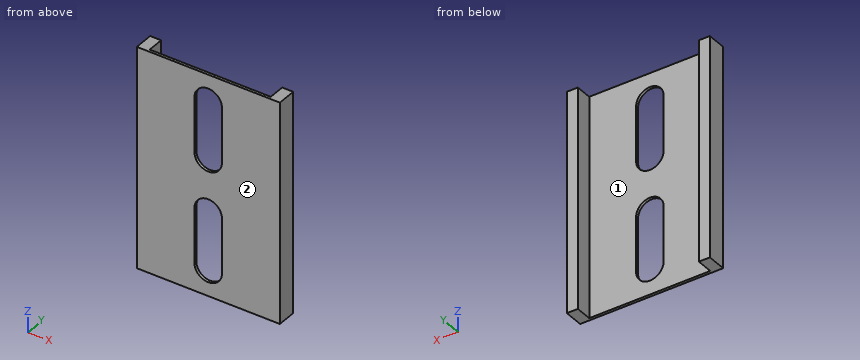
from build123d import *

# Parameters (mm, degrees)
F1_DEPTH = 400
F3_DEPTH = 25


with BuildPart() as f1:
    # F0 (on Top) → F1 (new body)
    with BuildSketch(Plane.XY):
        Polygon((-130, 17.5), (-130, -17.5), (130, -17.5), (130, 17.5), (110, 17.5), (110, -12.5), (-110, -12.5), (-110, 17.5), align=None)
    extrude(amount=F1_DEPTH)

    # F2 (on face) → F3 (cut)
    with BuildSketch(Plane.XZ.offset(17.5)):
        with BuildLine():
            Line((-25.221969, 350), (-25.221969, 250))
            ThreePointArc((-25.221969, 250), (-0.221969, 225), (24.778031, 250))
            Line((24.778031, 250), (24.778031, 350))
            ThreePointArc((24.778031, 350), (-0.221969, 375), (-25.221969, 350))
        make_face()
        with BuildLine():
            Line((24.778031, 50), (24.778031, 150))
            ThreePointArc((24.778031, 150), (-0.221969, 175), (-25.221969, 150))
            Line((-25.221969, 150), (-25.221969, 50))
            ThreePointArc((-25.221969, 50), (-0.221969, 25), (24.778031, 50))
        make_face()
    extrude(amount=-F3_DEPTH, mode=Mode.SUBTRACT)


solid = f1.part
Input: part model. Units: mm. Frame: model coordinates. Face numbers are marked on the shaded views. Coordinates: 2 decimals unless noted, no trailing zeros. Order: outer loops, then holes, each group sorted by start corner. A loop starts at its lowest first (then second) coordinate and runs counter-clockwise, first axis right, second up.
1. Cut plane B-B, the plane y = -2.5. Return loops of the section in (x, z), plus the area to 3 significant figures.
Checked values:
outline: (-130, 0) - (-110, 0) - (-110, 400) - (-130, 400) - close; (110, 0) - (130, 0) - (130, 400) - (110, 400) - close
area: 16,000 mm2
2. Contact query for a flat-ended pin moving along its axis: P1, Ø1, axis at x = 63.5, z = 277, coming from the +Y side. Output: stop coordinate, or through.
Checked values:
P1: stops at y = -12.5
3. Draft query along X for the marked faces 1 and 2. Return one class per face: +X half, -X half, draft (parallel to the pull), parting line (faces both ways), or undercut.
Checked values:
face 1: undercut
face 2: draft
4. Cut plane A-A, the plane z = 139. Return loops of the section in (x, y), plus the area to 3 significant figures.
Checked values:
outline: (-130, -17.5) - (-25.22, -17.5) - (-25.22, -12.5) - (-110, -12.5) - (-110, 17.5) - (-130, 17.5) - close; (24.78, -17.5) - (130, -17.5) - (130, 17.5) - (110, 17.5) - (110, -12.5) - (24.78, -12.5) - close
area: 2,250 mm2
5. Cut plane C-C, the plane x = 8. Return loops of the section in (y, z), plus the area to 3 significant figures.
Checked values:
outline: (-17.5, 0) - (-12.5, 0) - (-12.5, 26.39) - (-17.5, 26.39) - close; (-17.5, 173.61) - (-12.5, 173.61) - (-12.5, 226.39) - (-17.5, 226.39) - close; (-17.5, 373.61) - (-12.5, 373.61) - (-12.5, 400) - (-17.5, 400) - close
area: 528 mm2
6. Cut plane D-D, the plane z = 243. Return loops of the section in (x, y), plus the area to 3 significant figures.
Checked values:
outline: (-130, -17.5) - (-24.22, -17.5) - (-24.22, -12.5) - (-110, -12.5) - (-110, 17.5) - (-130, 17.5) - close; (23.78, -17.5) - (130, -17.5) - (130, 17.5) - (110, 17.5) - (110, -12.5) - (23.78, -12.5) - close
area: 2,260 mm2
7. Ray query, line 1 along X through (y, z) = (9.5, 36); line 2 along X through (y, z) = (-15, 298); line 3 along Y through (x, z) = (-82.5, 380.5). Return the intervals inside material, ascending.
Checked values:
line 1: x = -130 to -110, 110 to 130
line 2: x = -130 to -25.22, 24.78 to 130
line 3: y = -17.5 to -12.5
